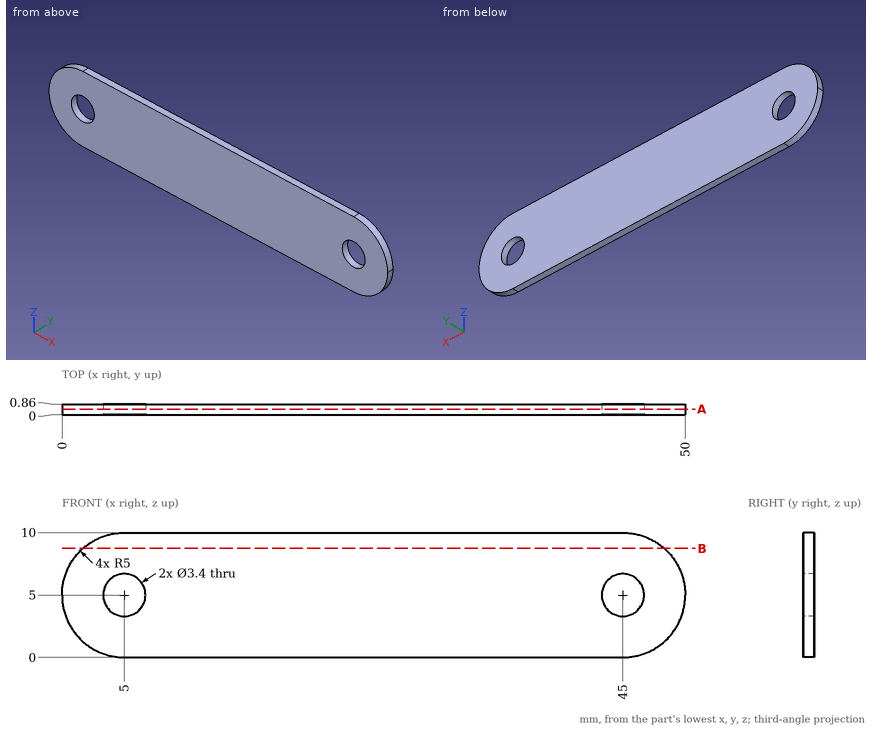
Study the drawing (mm; zero at the part's minimum x, y, z) and answer. Coordinates: 2 decimals unless noted, no trailing zeros. Write each loop counter-clockwise with the first axis right and the second up, starting at its lowest first coordinate (ties: lowest second). Pieces come first, ordered by that corner, then holes. Notation, with made-up numbers: (-10, 89.5) - (2, 89.5) arc R17 ccw to (2, 114.5) - close; hole circle Ø10 at (-20.5, 88). An arc over 180 degrees is marked (long way). Return JSON: item names as keys, results as strings. Group by question number.
1. A cutting plane is placed at A-A, the plane y = 0.45. Give the number of separate pieces and of enclosed holes in the cut face, plus the area to 3 significant figures.
2. A cutting plane is placed at B-B, the plane z = 8.75. Determine the outline of the cut face in (x, y).
3. Straight lines are drawn through the part: L1, parallel to Z at x = 5, y = 0.65; L2, parallel to Z at x = 44.5, y = 0.5 (1 decimal); L3, parallel to X at y = 0.6, z = 6 (1 decimal). For each, find the intervals that lie inside material, in ascending order.
Ans:
{
 "1": {"separate pieces": "1", "enclosed holes": "2", "area": "460 mm²"},
 "2": {"outline": "(1.69, 0) - (48.31, 0) - (48.31, 0.86) - (1.69, 0.86) - close"},
 "3": {"L1": "0 to 3.3, 6.7 to 10", "L2": "0 to 3.4, 6.6 to 10", "L3": "0.1 to 3.6, 6.4 to 43.6, 46.4 to 49.9"}
}
